Can you work these out from the model? Positions are in its coordinate system, mm. A direction names the side the tool comes from. Round coordinates to 2 decimals unless told otherwise and drop trailing zeros. Loops run counter-clockwise (first coordinate to the right, second up) from the corner with the lowest first, then second, coordinate; pieces in that order, holes last. Notation, with made-up numbers: (22.5, 86) -> (81.5, 86) arc R19 cw to (81.5, 112) -> close; hole circle Ø6 at (57.25, 88.25). An arc over 180 degrees is marked (long way). Write each question's results on one line, items separated by ' | '.
from build123d import *

# Parameters (mm, degrees)
F0_W     = 75
F0_H     = 50
F1_DEPTH = 5
F3_DEPTH = 10
F4_R     = 4
F5_R     = 1
F6_DEPTH = 7
F7_W     = 65
F7_H     = 40
F8_DEPTH = 10


with BuildPart() as f1:
    # F0 (on Top) → F1 (new body)
    with BuildSketch(Plane.XY):
        Rectangle(F0_W, F0_H)
    extrude(amount=F1_DEPTH)

    # F2 (on face) → F3 (join)
    with BuildSketch(Plane(origin=(0, 0, 0), x_dir=(1, 0, 0), z_dir=(0, 0, -1))):
        Polygon((37.5, 25), (-37.5, 25), (-37.5, -25), (-27.5, -25), (-27.5, -40), (27.5, -40), (27.5, -25), (37.5, -25), align=None)
    extrude(amount=F3_DEPTH)

    # F4
    f4_edges = [f1.edges().sort_by_distance(p)[0] for p in [
        (0, -25, 5),
        (37.5, 0, 5),
        (0, 25, 5),
        (-37.5, 0, 5),
        (27.5, 32.5, 0),
        (0, 40, 0),
        (-27.5, 32.5, 0),
    ]]
    fillet(f4_edges, radius=F4_R)

    # F5 (on face) → F6 (cut)
    with BuildSketch(Plane.XY):
        with Locations((-19.5, 30.5)):
            Circle(F5_R)
        with Locations((-4, 30.5)):
            Circle(F5_R)
        with Locations((4, 30.5)):
            Circle(F5_R)
        with Locations((19.5, 30.5)):
            Circle(F5_R)
    extrude(amount=-F6_DEPTH, mode=Mode.SUBTRACT)

    # F7 (on face) → F8 (cut)
    with BuildSketch(Plane.XY.offset(5)):
        Rectangle(F7_W, F7_H)
    extrude(amount=-F8_DEPTH, mode=Mode.SUBTRACT)


solid = f1.part
1. If we section it at C-C (y = -19): List the corners of the cut face in (x, z) for me, then the cut area to 3 significant figures.
Final values:
outline: (-37.5, -10) -> (37.5, -10) -> (37.5, 1) arc R4 ccw to (33.5, 5) -> (32.5, 5) -> (32.5, -5) -> (-32.5, -5) -> (-32.5, 5) -> (-33.5, 5) arc R4 ccw to (-37.5, 1) -> close | area: 468 mm2
2. If we section it at D-D (x = -4): List the corners of the cut face in (y, z) for me, then the cut area to 3 significant figures.
Final values:
outline: (-25, -10) -> (40, -10) -> (40, -4) arc R4 ccw to (36, 0) -> (31.5, 0) -> (31.5, -7) -> (29.5, -7) -> (29.5, 0) -> (25, 0) -> (25, 1) arc R4 ccw to (21, 5) -> (20, 5) -> (20, -5) -> (-20, -5) -> (-20, 5) -> (-21, 5) arc R4 ccw to (-25, 1) -> close | area: 476 mm2
3. Please list where these lines run through material, in increasing order: line 1 (Y direction, x = 21.5, z = -4.75); line 2 (Y direction, x = -19.5, z = -4.5); line 3 (X direction, y = 31, z = -5.5). Write a range as from..to.
Final values:
line 1: -25..-20, 20..40 | line 2: -25..-20, 20..29.5, 31.5..40 | line 3: -27.5..-20.37, -18.63..-4.87, -3.13..3.13, 4.87..18.63, 20.37..27.5
4. Will these pins go through, and if not, where does the flat tip stop? pin 1 (8 mm diameter, centred on y = 31.5, z = 3, fed in from +X); pin 2 (12 mm diameter, centred on x = 7.5, y = 29, fed in from +Z); pin 3 (1 mm diameter, centred on x = 20, y = 31, fed in from +Z).
Final values:
pin 1: x = 26.15 | pin 2: z = 4.46 | pin 3: z = 0
5. If we section it at B-B (z = -1): List the corners of the cut face in (x, y) for me, then the cut area to 3 significant figures.
Final values:
outline: (-37.5, -25) -> (37.5, -25) -> (37.5, 25) -> (26.15, 25) -> (26.15, 38.65) -> (-26.15, 38.65) -> (-26.15, 25) -> (-37.5, 25) -> close; hole (-32.5, -20) -> (32.5, -20) -> (32.5, 20) -> (-32.5, 20) -> close; hole circle Ø2 at (-19.5, 30.5); hole circle Ø2 at (-4, 30.5); hole circle Ø2 at (4, 30.5); hole circle Ø2 at (19.5, 30.5) | area: 1,850 mm2
6. If we section it at A-A (x = 8): List the corners of the cut face in (y, z) for me.
Final values:
outline: (-25, -10) -> (40, -10) -> (40, -4) arc R4 ccw to (36, 0) -> (25, 0) -> (25, 1) arc R4 ccw to (21, 5) -> (20, 5) -> (20, -5) -> (-20, -5) -> (-20, 5) -> (-21, 5) arc R4 ccw to (-25, 1) -> close
7. We'd pull the mould along Y, two halves only. Please class faces 1 (the face through (32.5, 0, 0)), 2 (the face through (-0.2, 25, 0.8)), 3 (the face through (-1, 7, -10)): pulls with the +Y half, pulls with the -Y half, needs draft (parallel to the pull), parting line crosses it, or undercut.
Final values:
face 1: undercut | face 2: pulls with the +Y half | face 3: needs draft
8. On a 3-axis mill with a long thin cutter (end or side, diameter ignored), from which of +Z, -Z, +X, -X, +Y, -Y can I reach the whole of each face in a straight line? I mean faces 4 (the face through (26.297, 32.395, -1.141)), 5 (the face through (-27.5, 32, -7)), 6 (the face through (27.5, 33, -7)), 7 (the face through (0, -20, 0)). Say none if no direction works.
Final values:
face 4: +Z, +X, +Y | face 5: +Z, -Z, -X, +Y | face 6: +Z, -Z, +X, +Y | face 7: +Z
